```python
from build123d import *

# Parameters (mm, degrees)
EXTRUDE_1_DEPTH          = 2
SKETCH_3_W               = 440.695596705
SKETCH_3_H               = 44.042045092
CUT_EXTRUDE_1_DEPTH      = 10
CUT_EXTRUDE_1_DEPTH_BACK = 10


with BuildPart() as part:
    # 스케치1 → 보스-돌출1 (new body)
    with BuildSketch(Plane.XY):
        Polygon((-221, 181), (-181, 221), (181, 221), (221, 181), (221, -181), (181, -221), (-181, -221), (-221, -181), align=None)
    extrude(amount=EXTRUDE_1_DEPTH)

    # 스케치3 → 컷-돌출1 (cut, two sides)
    with BuildSketch(Plane.XY) as cut_extrude_1_sk:
        with Locations((5.347798353, 230.521022546)):
            Rectangle(SKETCH_3_W, SKETCH_3_H)
    extrude(amount=CUT_EXTRUDE_1_DEPTH, mode=Mode.SUBTRACT)
    extrude(cut_extrude_1_sk.sketch, amount=-CUT_EXTRUDE_1_DEPTH_BACK, mode=Mode.SUBTRACT)


solid = part.part
```
Could you check a few things on this model? Use its own coordinates, in mm. Coordinates: 2 decimals unless noted, no trailing zeros. Write each loop counter-clockwise with the first axis right and the second up, starting at its lowest first coordinate (ties: lowest second). Pieces come first, ordered by that corner, then holes. Notation, with made-up numbers: (54.25, -3) -> (80.25, -3) arc R31 ccw to (80.25, 26) -> close; hole circle Ø5 at (38.5, 28). An arc over 180 degrees is marked (long way). Return JSON: item names as keys, results as strings.
(1) I need wall thicknesses on L1, parallel to Y at x = 182.5, z = 1.7; L2, parallel to X at y = -191, z = 1.15; L3, parallel to Y at x = 190.5, z = 1.35. Which ranges of each line are inside material? Lowest first, please.
Numbers:
{"L1": "y = -219.5 to 208.5", "L2": "x = -211 to 211", "L3": "y = -211.5 to 208.5"}
(2) Imagine slicing it at A-A, the plane y = -191. Please give me the cut outline in (x, z).
Numbers:
{"outline": "(-211, 0) -> (211, 0) -> (211, 2) -> (-211, 2) -> close"}
(3) Imagine slicing it at B-B, the plane x = -188. Please give me the cut outline in (y, z), then the cut area to 3 significant figures.
Numbers:
{"outline": "(-214, 0) -> (208.5, 0) -> (208.5, 2) -> (-214, 2) -> close", "area": "845 mm2"}
(4) I'm going to push a flat-ended pin straight in: pin 1 (1.5 mm diameter, centred on x = 8, y = -76.5, fed in from -Z). Where does the tip first touch, or does it pass through?
Numbers:
{"pin 1": "stops at z = 0"}
